Check sheet for the modelled part. Datum: model origin and axes. Units: mm. A direction names the side the tool comes from. Give positions to 0.01 mm unless a question says otherwise; leave off trailing zeros. Loops run counter-clockwise (first coordinate to the right, second up) from the corner with the lowest first, then second, coordinate; pieces in that order, holes last. Notation, with made-up numbers: M -31.5,33 L -22.5,33 A35 cw -22.5,71 Z; hole C 48,27.5 d8. An arc over 180 degrees is marked long. Write each question's results on one line, items separated by ' | '. Start each with the question number.
1. Tool access check on faces 1 (the flat face through (2, 3, 0)), 2 (the flat face through (8.2, 13, 0)). Record the directions out of +Z, -Z, +X, -X, +Y, -Y that give a thin tool (end or side, any length) a straight path to the whole face; none if there is none.
2. Go/stop test with flat-tipped pins: pin 1 (8 mm diameter, centred on x = 0, z = -1.5, fed in from +Y); pin 2 (3 mm diameter, centred on y = 9, z = 6.5, fed in from -X); pin 3 (2 mm diameter, centred on x = 7, y = 6.5, fed in from -Z). Record where each tip stops, or that it passes through.
3. Sectioned sample at C-C on y = 2. Record the cut outline in (x, z).
4. Material ranges on line 1 along Y through (x, z) = (8.35, 0); line 2 along X through (y, z) = (1.4, 0); line 3 along X through (y, z) = (5, 0), recorded low to high.
5. Sectioned sample at B-B on z = 0. Record the cut outline in (x, y), and give its area (3 significant figures).
6. Sectioned sample at D-D on z = 2.5. Record the cut outline in (x, y).
7. Sectioned sample at A-A on x = 0. Record the cut outline in (y, z).
8. Draft check along X on faces 3 (the cylindrical face through (-7.81, 7.93, -1.73)), 4 (the cylindrical face through (8.942, 6.425, -1.386)), 5 (the cylindrical face through (-1.71, 1.52, -0.38)), 6 (the cylindrical face through (-9.76, 6.41, -2.17)). Enter one of: pulls with the +X half, pulls with the -X half, needs draft (parallel to the pull), parting line crosses it, or undercut.
```python
from build123d import *

# Parameters (mm, degrees)
SKETCH1_R           = 10
BOSS_EXTRUDE1_DEPTH = 3
SKETCH2_R           = 1.75
CUT_EXTRUDE1_DEPTH  = 3
SKETCH3_R           = 10
SKETCH3_R_2         = 8
BOSS_EXTRUDE2_DEPTH = 10
SKETCH4_R           = 1.5
CUT_EXTRUDE2_DEPTH  = 5


with BuildPart() as part:
    # Sketch1 → Boss-Extrude1 (new body)
    with BuildSketch(Plane(origin=(0, 0, 0), x_dir=(1, 0, 0), z_dir=(0, 1, 0))):
        with Locations(Location((0, 0, 0), (0, 0, 270))):
            Circle(SKETCH1_R)
    extrude(amount=BOSS_EXTRUDE1_DEPTH)

    # Sketch2 → Cut-Extrude1 (cut)
    with BuildSketch(Plane(origin=(0, 3, 0), x_dir=(1, 0, 0), z_dir=(0, 1, 0))):
        with Locations(Location((0, 0, 0), (0, 0, 270))):
            Circle(SKETCH2_R)
    extrude(amount=-CUT_EXTRUDE1_DEPTH, mode=Mode.SUBTRACT)

    # Sketch3 → Boss-Extrude2 (add)
    with BuildSketch(Plane(origin=(0, 3, 0), x_dir=(1, 0, 0), z_dir=(0, 1, 0))):
        with Locations(Location((0, 0, 0), (0, 0, 270))):
            Circle(SKETCH3_R)
        with Locations(Location((0, 0, 0), (0, 0, 270))):
            Circle(SKETCH3_R_2, mode=Mode.SUBTRACT)
    extrude(amount=BOSS_EXTRUDE2_DEPTH)

    # Sketch4 → Cut-Extrude2 (cut)
    with BuildSketch(Plane(origin=(10, 0, 0), x_dir=(0, 0, -1), z_dir=(1, 0, 0))):
        with Locations((0, 7)):
            Circle(SKETCH4_R)
    extrude(amount=-CUT_EXTRUDE2_DEPTH, mode=Mode.SUBTRACT)


solid = part.part
```
Output values:
1) face 1: +Y | face 2: +Z, -Z, +X, -X, +Y
2) pin 1: y = 3 | pin 2: x = -8.66 | pin 3: z = -8
3) outline: C 0,0 d20; hole C 0,0 d3.5
4) line 1: 0 to 5.5, 8.5 to 13 | line 2: -10 to -1.75, 1.75 to 10 | line 3: -10 to -8, 8 to 10
5) outline: M -10,0 L -1.75,0 L -1.75,3 L -8,3 L -8,13 L -10,13 Z; M 1.75,0 L 10,0 L 10,5.5 L 8,5.5 L 8,3 L 1.75,3 Z; M 8,8.5 L 10,8.5 L 10,13 L 8,13 Z | area: 83.5 mm2
6) outline: M -9.68,0 L 9.68,0 L 9.68,13 L 7.6,13 L 7.6,3 L -7.6,3 L -7.6,13 L -9.68,13 Z
7) outline: M 0,-10 L 13,-10 L 13,-8 L 3,-8 L 3,-1.75 L 0,-1.75 Z; M 0,1.75 L 3,1.75 L 3,8 L 13,8 L 13,10 L 0,10 Z
8) face 3: undercut | face 4: needs draft | face 5: undercut | face 6: parting line crosses it
